Geometry check sheet. Reference: the model listing, model coordinates, mm. Face numbers are marked on the shaded views. A direction names the side the tool comes from. Give positions to 0.01 mm unless a question says otherwise; leave off trailing zeros. Write each loop counter-clockwise with the first axis right and the second up, starting at its lowest first coordinate (ties: lowest second). Pieces come first, ordered by that corner, then holes. Notation, with made-up numbers: M 52,45.5 L 70,45.5 A30 ccw 70,82.5 Z; hole C 1,-29.5 d9. An arc over 180 degrees is marked long. One line per item, written item: value. Start each with the question number.
1. Cross-section at D-D on z = -9. Record the cut outline in (x, y), then the cut area to 3 significant figures.
2. Scan lines: line 1 (Z direction, x = -4, y = 1.1); line 2 (X direction, y = 1.55, z = -2.5); line 3 (X direction, y = 4.25, z = 0). Record each from-to range of solid material in increasing order.
3. Gauge pin test, flat ends, axial feed: pin 1 (2.5 mm diameter, centred on x = -5.5, z = 8, fed in from -Y); pin 2 (1.5 mm diameter, centred on x = 0, y = 3, fed in from -Z); pin 3 (2 mm diameter, centred on x = 0, z = 0, fed in from +Y); pin 4 (0.7 mm diameter, centred on x = -1.5, z = 0, fed in from +Y). Record the tip position at first contact, or that the pin passes through.
4. Cross-section at B-B on y = 2.4. Record the cut outline in (x, z).
5. Release check for a two-part mould opening along X. For the marked faces 1, 2 and 3 record: pulls with the +X half, pulls with the -X half, needs draft (parallel to the pull), parting line crosses it, or undercut.
6. Tool access check on the marked faces 4, 5 and 6. Record the directions out of +Z, -Z, +X, -X, +Y, -Y that give a thin tool (end or side, any length) a straight path to the whole face; none if there is none.
7. Cross-section at C-C on x = -4. Record the cut outline in (y, z), then the cut area to 3 significant figures.
8. Cross-section at A-A on y = 5. Record the cut outline in (x, z), then the cut area to 3 significant figures.
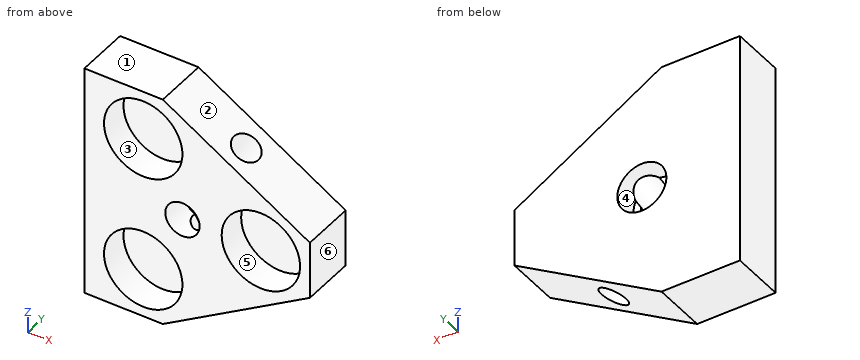
Autodesk Inventor part; units mm, degrees
ref_plane "YZ Plane" through (0, 0, 0) normal (1, 0, 0) x (0, 1, 0)
ref_plane "XZ Plane" through (0, 0, 0) normal (0, 1, 0) x (-1, 0, 0)
ref_plane "XY Plane" through (0, 0, 0) normal (0, 0, 1) x (1, 0, 0)
sketch "Sketch1" plane through (0, 0, 0) normal (0, 1, 0) x (-1, 0, 0)
  line L0 (-13, -11.9282) -> (10, -11.9282)
  line L1 (10, -11.9282) -> (10, 11.9282)
  line L2 (10, 11.9282) -> (-13, 11.9282)
  line L3 (-13, 11.9282) -> (-13, -11.9282)
  circle A0 centre (-8, 0) radius 4
  circle A1 centre (4, -6.9282) radius 4
  circle A2 centre (4, 6.9282) radius 4
  circle A3 centre (0, 0) radius 8 construction
  circle A4 centre (0, 0) radius 1.75
  dimension "d11" = 16
  dimension "d2" = 8
  dimension "d6" = 360
  dimension "d8" = 6
  dimension "d9" = 5
  dimension "d12" = 5
  dimension "d13" = 5
  dimension "d35" = 3.5
extrude "Extrusion1" add sketch "Sketch1" along normal blind 3
sketch "Sketch2" plane through (0, 3, 0) normal (0, 1, 0) x (1, 0, 0)
  circle A0 centre (-4, -6.9282) radius 4
  circle A1 centre (-4, 6.9282) radius 4
  circle A2 centre (8, 0) radius 4
  line L0 (13, 11.9282) -> (-10, 11.9282)
  line L1 (-10, 11.9282) -> (-10, -11.9282)
  line L2 (-10, -11.9282) -> (13, -11.9282)
  line L3 (13, -11.9282) -> (13, 11.9282)
  circle A3 centre (0, 0) radius 2.5
  dimension "d16" = 5
extrude "Extrusion2" add sketch "Sketch2" along normal blind 2.5 contours A0 | A1 | A2 | L3 L2 L1 L0
sketch "Sketch3" plane through (0, 0, 0) normal (0, -1, 0) x (1, 0, 0)
  circle A0 centre (-4, 6.9282) radius 4
  circle A1 centre (-4, -6.9282) radius 4
  circle A2 centre (8, 0) radius 4
  line L0 (13, -11.9282) -> (-10, -11.9282)
  line L1 (13, 11.9282) -> (13, -11.9282)
  line L2 (-10, 11.9282) -> (13, 11.9282)
  line L3 (-10, -11.9282) -> (-10, 11.9282) construction
  line L4 (-2, 11.9282) -> (13, 2.9282)
  line L5 (13, 11.9282) -> (13, -11.9282)
  line L6 (13, -2.9282) -> (-2, -11.9282)
  point P0 (0, 0)
  dimension "d19" = 9
  dimension "d20" = 9
  dimension "d21" = 15
  dimension "d22" = 15
extrude "Extrusion3" cut sketch "Sketch3" against normal through all contours L4 L2 L1 | L0 L6 L1
sketch "Skizze10" plane through (-2, 0, 11.9282) normal (0.5145, 0, 0.8575) x (0.8575, 0, -0.5145)
  line L0 (9.602, 0) -> (6.102, 0)
  line L1 (9.602, 0) -> (9.602, 3)
  line L2 (6.102, 0) -> (6.102, 3)
  circle A0 centre (7.852, 2.6816) radius 1.45
  point P0 (7.852, 0)
  dimension "d42" = 2.9
extrude "Extrusion9" cut sketch "Skizze10" against normal up to surface
ref_plane "Arbeitsebene1" through (-10, 0, 0) normal (0, 0, 1) x (1, 0, 0)
mirror "Spiegeln1" about plane through (-10, 0, 0) normal (0, 0, 1) of "Extrusion9"
equation "\"d12\" = d9"
equation "\"d13\" = d9"
equation "\"d43\" = d42"
properties part number "30_Cube_Z_Focus_Drylin_NEMA_slide_part1"
Report:
1. outline: M -10,0 L -7.42,0 L -7.42,3 L -0.58,3 L -0.58,0 L 2.88,0 L 2.88,5.5 L -10,5.5 Z
1. area: 50.3 mm^2
2. line 1: z = -11.93 to -10.93, -2.93 to 2.93, 10.93 to 11.93
2. line 2: x = -10 to 0.44, 2.56 to 4.88, 11.12 to 13
2. line 3: x = -10 to -2.5, 2.5 to 13
3. pin 1: stops at y = 3
3. pin 2: stops at z = -11.18
3. pin 3: passes through
3. pin 4: stops at y = 3
4. outline: M -10,-11.93 L -2,-11.93 L 3.51,-8.62 L -0.7,-1.61 A1.75 cw -0.7,1.61 L 3.51,8.62 L -2,11.93 L -10,11.93 Z; M 1.74,-0.14 L 5.95,-7.16 L 13,-2.93 L 13,2.93 L 5.95,7.16 L 1.74,0.14 A1.75 cw Z; hole C -4,-6.93 d8; hole C -4,6.93 d8; hole C 8,0 d8
5. face 1: needs draft
5. face 2: pulls with the +X half
5. face 3: undercut
6. face 4: +Y
6. face 5: -Y
6. face 6: +Z, -Z, +X, +Y, -Y
7. outline: M 0,-11.93 L 5.5,-11.93 L 5.5,11.93 L 0,11.93 L 0,10.93 L 3,10.93 L 3,2.93 L 0,2.93 L 0,-2.93 L 3,-2.93 L 3,-10.93 L 0,-10.93 Z
7. area: 83.2 mm^2
8. outline: M -10,-11.93 L -2,-11.93 L 13,-2.93 L 13,2.93 L -2,11.93 L -10,11.93 Z; hole C 0,0 d5
8. area: 394 mm^2
